```python
from build123d import *

# Parameters (mm, degrees)
F0_R      = 40
F1_DEPTH  = 2.5
F2_R      = 12
F3_DEPTH  = 3
F4_R      = 2
F5_DEPTH  = 25
F6_R      = 3.25
F7_DEPTH  = 25
F9_R      = 2
F10_DEPTH = 25


with BuildPart() as f1:
    # F0 (on Top) → F1 (new body)
    with BuildSketch(Plane.XY):
        Circle(F0_R)
    extrude(amount=F1_DEPTH)

    # F2 (on face) → F3 (join)
    with BuildSketch(Plane.XY.offset(2.5)):
        Circle(F2_R)
    extrude(amount=F3_DEPTH)

    # F4 (on face) → F5 (cut)
    with BuildSketch(Plane.XY.offset(5.5)):
        with Locations((-7.3, 0)):
            Circle(F4_R)
        with Locations((7.3, 0)):
            Circle(F4_R)
        with Locations((0, -7.3)):
            Circle(F4_R)
    extrude(amount=-F5_DEPTH, mode=Mode.SUBTRACT)

    # F6 (on face) → F7 (cut)
    with BuildSketch(Plane.XY.offset(5.5)):
        Circle(F6_R)
    extrude(amount=-F7_DEPTH, mode=Mode.SUBTRACT)

    # F9 (on face) → F10 (cut)
    with BuildSketch(Plane.XY.offset(2.5)):
        with Locations((21.9, 0)):
            Circle(F9_R)
        with Locations((16.9, 11.5)):
            Circle(F9_R)
        with Locations((26.9, -11.5)):
            Circle(F9_R)
        with Locations((-26.9, 11.5)):
            Circle(F9_R)
        with Locations((-21.9, 0)):
            Circle(F9_R)
        with Locations((-16.9, -11.5)):
            Circle(F9_R)
    extrude(amount=-F10_DEPTH, mode=Mode.SUBTRACT)


solid = f1.part
```
Could you check a few things on this model? Use its own coordinates, in mm. A direction names the side the tool comes from. Coordinates: 2 decimals unless noted, no trailing zeros. Order: outer loops, then holes, each group sorted by start corner. A loop starts at its lowest first (then second) coordinate and runs counter-clockwise, first axis right, second up. Notation, with made-up numbers: M 80,80.5 L 91,80.5 A24 cw 91,101.5 Z; hole C -12,-15 d6. An arc over 180 degrees is marked long. Use one line per item in the form item = value. Start each with the question number.
1. Please list where these lines run through material, in increasing order: line 1 (Y direction, x = -21.9, z = 1.85); line 2 (Y direction, x = 26.9, z = 1.1); line 3 (X direction, y = -3, z = 1.7).
2. Suppose I cut it at B-B on y = 0. Write out the boundary of the cut face in (x, z), then the cut area to 3 significant figures.
3. On a 3-axis mill with a long thin cutter (end or side, diameter ignored), from which of +Z, -Z, +X, -X, +Y, -Y can I reach the whole of each face in a straight line? I mean faces 1 (the cylindrical face through (24.902, -11.412, 1.268)), 2 (the cylindrical face through (-11.99, 0.53, 3.98)). Say none if no direction works.
4. Suppose I cut it at D-D on x = -21.9. Write out the boundary of the cut face in (y, z).
5. Suppose I cut it at C-C on z = 3.4. Write out the boundary of the cut face in (x, y).
6. For pin 1 (3 mm diameter, centred on x = 21.9, y = 0, fed in from -Z); pin 2 (6.5 mm diameter, centred on x = -16.9, y = -11.5, fed in from +Z); pin 3 (2 mm diameter, centred on y = -21, z = 2.5, fed in from -X), each with a flat end and sliding along its axis, tell me the tip position at first contact or that it passes through.
7. Suppose I cut it at A-A on x = 0. Write out the boundary of the cut face in (y, z), then the cut area to 3 significant figures.
Geometry says:
q1.line_1 = -33.47 to -2, 2 to 33.47
q1.line_2 = -29.6 to -13.5, -9.5 to 29.6
q1.line_3 = -39.89 to -1.25, 1.25 to 39.89
q2.outline = M -40,0 L -23.9,0 L -23.9,2.5 L -40,2.5 Z; M -19.9,0 L -9.3,0 L -9.3,5.5 L -12,5.5 L -12,2.5 L -19.9,2.5 Z; M -5.3,0 L -3.25,0 L -3.25,5.5 L -5.3,5.5 Z; M 3.25,0 L 5.3,0 L 5.3,5.5 L 3.25,5.5 Z; M 9.3,0 L 19.9,0 L 19.9,2.5 L 12,2.5 L 12,5.5 L 9.3,5.5 Z; M 23.9,0 L 40,0 L 40,2.5 L 23.9,2.5 Z
q2.area = 172 mm^2
q3.face_1 = +Z, -Z
q3.face_2 = +Z
q4.outline = M -33.47,0 L -2,0 L -2,2.5 L -33.47,2.5 Z; M 2,0 L 33.47,0 L 33.47,2.5 L 2,2.5 Z
q5.outline = C 0,0 d24; hole C -7.3,0 d4; hole C 0,0 d6.5; hole C 0,-7.3 d4; hole C 7.3,0 d4
q6.pin_1 = through
q6.pin_2 = 2.5
q6.pin_3 = -34.64
q7.outline = M -40,0 L -9.3,0 L -9.3,5.5 L -12,5.5 L -12,2.5 L -40,2.5 Z; M -5.3,0 L -3.25,0 L -3.25,5.5 L -5.3,5.5 Z; M 3.25,0 L 40,0 L 40,2.5 L 12,2.5 L 12,5.5 L 3.25,5.5 Z
q7.area = 214 mm^2
